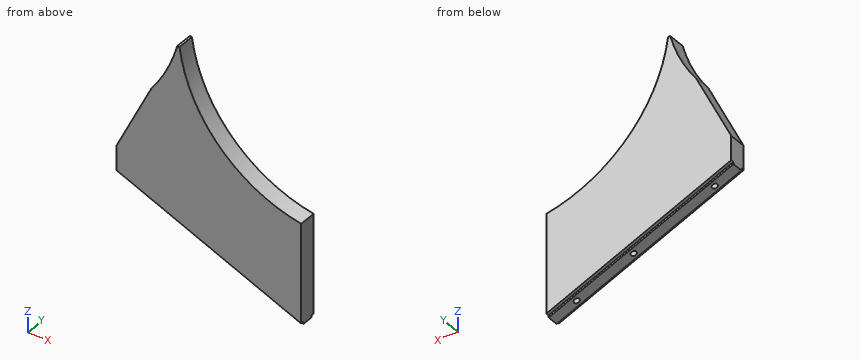
```python
from build123d import *

# Parameters (mm, degrees)
F1_DEPTH = 25.4
F3_D     = 7.9375
F3_DEPTH = 25.4
F3_TIP   = 2.3846655818
F5_DEPTH = 4.572
F7_DEPTH = 4.572


with BuildPart() as f1:
    # F0 (on Front) → F1 (new body)
    with BuildSketch(Plane.XZ):
        with BuildLine():
            ThreePointArc((266.7, 32.3849999569), (149.0538498691, 95.5862080763), (91.0917861403, 215.8999999569))
            Line((91.0917861403, 215.8999999569), (87.9167861403, 215.8999999569))
            ThreePointArc((87.9167861403, 215.8999999569), (72.9914115298, 176.3989748545), (50.662743739, 140.5586569695))
            Line((50.662743739, 140.5586569695), (0, 38.0999999569))
            Line((0, 38.0999999569), (0, -4.31e-08))
            Line((0, -4.31e-08), (266.7, -113.7158000431))
            Line((266.7, -113.7158000431), (266.7, -4.31e-08))
            Line((266.7, -4.31e-08), (266.7, 32.3849999569))
        make_face()
    extrude(amount=F1_DEPTH)

    # F3
    with Locations(Plane(origin=(-1.56e-08, 0, -3.65e-08), x_dir=(0.9198730081, 0, -0.3922163293), z_dir=(-0.3922163293, 0, -0.9198730081))):
        with Locations((35.4106249365, 12.7), (162.7154249365, 12.7), (252.0980249365, 12.7)):
            Hole(F3_D / 2, depth=F3_DEPTH)
            with Locations((0, 0, -(F3_DEPTH + F3_TIP / 2))):  # 118° drill point
                Cone(0, F3_D / 2, F3_TIP, mode=Mode.SUBTRACT)

    # F4 (on face) → F5 (cut)
    with BuildSketch(Plane.XZ.offset(25.4)):
        Polygon((0, 3.1749999569), (0, -4.31e-08), (266.7, -113.7158000431), (266.7, -110.5408000431), align=None)
    extrude(amount=-F5_DEPTH, mode=Mode.SUBTRACT)

    # F6 (on face) → F7 (cut)
    with BuildSketch(Plane(origin=(0, 0, 0), x_dir=(-1, 0, 0), z_dir=(0, 1, 0))):
        Polygon((-266.7, -110.5408000431), (-266.7, -113.7158000431), (0, -4.31e-08), (0, 3.1749999569), align=None)
    extrude(amount=-F7_DEPTH, mode=Mode.SUBTRACT)


solid = f1.part
```
Can you work these out from the model? Positions are in its coordinate system, mm. Coordinates: 2 decimals unless noted, no trailing zeros. Loops run counter-clockwise (first coordinate to the right, second up) from the corner with the lowest first, then second, coordinate; pieces in that order, holes last. Notation, with made-up numbers: (-10, -35.5) - (41, -35.5) arc R13 cw to (41, -16.5) - close; hole circle Ø10 at (54, -26). An arc over 180 degrees is marked (long way). Answer as CSV lines item,"result". Start each with the question number.
1) Suppose I cut it at C-C (x = 134). Please give me the cut outline in (y, z), plus the area to 3 significant figures.
2) Suppose I cut it at A-A (x = 106). Please give me the cut outline in (y, z).
3) Suppose I cut it at D-D (z = 193). Please give me the cut outline in (x, y).
4) Suppose I cut it at B-B (z = 158). Please give me the cut outline in (x, y).
5) For pin 1 (2 mm diameter, centred on x = 40, y = -5, fed in from -Z); pin 2 (2 mm diameter, centred on y = -18.5, z = 138, fed in from -X); pin 3 (12 mm diameter, centred on x = 41.5, y = -15.5, fed in from -Z), each with a flat end and sliding along its axis, tell me the tip position at first contact or that it passes through.
6) I need wall thicknesses on line 1 (X direction, y = -6.25, z = 94.5); line 2 (Z direction, x = 37, y = -12.5); line 3 (Z direction, x = 24, y = -7). Which ranges of each line are inside material? Lowest first, please. Write a range as from..to.
Check result:
1,outline,"(-25.4, -53.96) - (-20.83, -53.96) - (-20.83, -57.14) - (-4.57, -57.14) - (-4.57, -53.96) - (0, -53.96) - (0, 113.11) - (-25.4, 113.11) - close"
1,area,"4,300 mm²"
2,outline,"(-25.4, -42.02) - (-20.83, -42.02) - (-20.83, -45.2) - (-4.57, -45.2) - (-4.57, -42.02) - (0, -42.02) - (0, 161.22) - (-25.4, 161.22) - close"
3,outline,"(80.35, -25.4) - (95.46, -25.4) - (95.46, 0) - (80.35, 0) - close"
4,outline,"(62.75, -25.4) - (107.38, -25.4) - (107.38, 0) - (62.75, 0) - close"
5,pin 1,"stops at z = -17.48"
5,pin 2,"stops at x = 48.9"
5,pin 3,"stops at z = -20.25"
6,line 1,"x = 27.89..150.1"
6,line 2,"z = -15.78..-13.61, 6.6..112.93"
6,line 3,"z = -10.23..86.64"
